Autodesk Fusion 360 part; units mm, degrees
sketch "草图1" plane through (0, 0, 0) normal (0, 0, 1) x (1, 0, 0)
  circle A0 centre (0, 0) radius 14.1
  line L0 (0, 9.064) -> (-7.85, -4.5326)
  line L1 (-7.85, -4.5326) -> (7.85, -4.5326)
  line L2 (7.85, -4.5326) -> (0, 9.064)
  line L3 (0, 9.064) -> (15.7, 9.064) construction
  circle A1 centre (0, 9.064) radius 1.5
  circle A2 centre (-7.85, -4.5326) radius 1.5
  circle A3 centre (7.85, -4.5326) radius 1.5
  point P0 (0, -0.0004)
  dimension "d1" = 28.2
  dimension "d2" = 15.7
  dimension "d3" = 120
  dimension "d4" = 9.064
  dimension "d5" = 3
  dimension "d6" = 3
  dimension "d7" = 3
extrude "拉伸1" add sketch "草图1" along normal blind 2 contours A0 | L0 L1 L2 A1 A2 A3
sketch "草图2" plane through (0, 0, 2) normal (0, 0, 1) x (-1, 0, 0)
  circle A0 centre (7.85, 4.5326) radius 1.5
  circle A1 centre (-7.85, 4.5326) radius 1.5
  circle A2 centre (0, -9.064) radius 1.5
  circle A3 centre (0, 0) radius 14.1
  circle A4 centre (0, 0) radius 2.2
  circle A5 centre (0, 0) radius 12
  circle A6 centre (0, 0) radius 4.2
  line L0 (0, 0) -> (4.5287, -11.1127)
  line L1 (0, 0) -> (11.7731, 2.3225)
  line L2 (0, 0) -> (7.3595, 9.4783)
  line L3 (0, 0) -> (-7.8979, 9.0345)
  line L4 (0, 0) -> (-11.8882, 1.6344)
  line L5 (0, 0) -> (-3.8752, -11.3571)
  dimension "d10" = 4.4
  dimension "d13" = 24
  dimension "d14" = 8.4
  dimension "d16" = 360
extrude "拉伸2" cut sketch "草图2" against normal blind 8 contours A4 L0 L1 | A4 L1 L2 | A4 L0 L5 | A4 L2 L3 | A4 L3 L4 | A4 L4 L5 | A5 A6 L0 L1 | A5 A6 L2 L3 | A5 A6 L4 L5
fillet "圆角1" radius 3 12 edges at (-1.585, 3.8894, 1) (-4.1206, -0.8129, 1) (-2.5758, -3.3174, 1) (2.7643, -3.1621, 1) (4.1609, -0.572, 1) (1.3563, 3.975, 1) (3.8752, 11.3571, 1) (11.8882, -1.6344, 1) (-4.5287, 11.1127, 1) (-11.7731, -2.3225, 1) (-7.3595, -9.4783, 1) (7.8979, -9.0345, 1)
Geometry check sheet. Reference: the model listing, model coordinates, mm. Give positions to 0.01 mm unless a question says otherwise; leave off trailing zeros. Write each loop counter-clockwise with the first axis right and the second up, starting at its lowest first coordinate (ties: lowest second). Pieces come first, ordered by that corner, then holes. Notation, with made-up numbers: (53.25, 11.5) -> (64.25, 11.5) arc R12 ccw to (64.25, 15.5) -> close; hole circle Ø3 at (56, 17.25). An arc over 180 degrees is marked (long way). One line per question, with ' | ' between items.
Item 1: Depth check by flat-ended pin: pin 1 (1 mm diameter, centred on y = -6, z = 1, fed in from -X); pin 2 (1.8 mm diameter, centred on x = 0, y = 9.064, fed in from +Z). Enter the tip coordinate at first touch or a pass-through.
Determined:
pin 1: x = -12.98 | pin 2: through
Item 2: Scan lines: line 1 along Y through (x, z) = (0, 0.4); line 2 along Y through (x, z) = (3, 0.95); line 3 along Y through (x, z) = (-7.85, 0.6). Record each from-to range of solid material in increasing order.
Determined:
line 1: -14.1 to -12, -4.2 to -2.2, 2.2 to 7.56, 10.56 to 14.1 | line 2: -13.78 to -11.62, -4.06 to 2.94, 8.59 to 13.78 | line 3: -11.71 to -6.03, -3.03 to -1.55, 9.07 to 11.71
Item 3: Sectioned sample at C-C, the plane z = 1.7. State how many separate pieces and enclosed holes the cut face has, plus the area to 3 significant figures.
Determined:
separate pieces: 1 | enclosed holes: 7 | area: 351 mm^2
Item 4: Sectioned sample at D-D, the plane x = 7.85. Record the boundary of the cut face in (y, z), plus the area to 3 significant figures.
Determined:
outline: (-11.71, 0) -> (-6.03, 0) -> (-6.03, 2) -> (-11.71, 2) -> close; (-3.03, 0) -> (-1.08, 0) -> (-1.08, 2) -> (-3.03, 2) -> close; (9.08, 0) -> (11.71, 0) -> (11.71, 2) -> (9.08, 2) -> close | area: 20.5 mm^2
Item 5: Sectioned sample at B-B, the plane y = 4. Record the boundary of the cut face in (x, z), plus the area to 3 significant figures.
Determined:
outline: (-13.52, 0) -> (-11.31, 0) -> (-11.31, 2) -> (-13.52, 2) -> close; (-2.4, 0) -> (2.21, 0) -> (2.21, 2) -> (-2.4, 2) -> close; (11.31, 0) -> (13.52, 0) -> (13.52, 2) -> (11.31, 2) -> close | area: 18.0 mm^2
Item 6: Sectioned sample at A-A, the plane x = 0. Record the boundary of the cut face in (y, z), plus the area to 3 significant figures.
Determined:
outline: (-14.1, 0) -> (-12, 0) -> (-12, 2) -> (-14.1, 2) -> close; (-4.2, 0) -> (-2.2, 0) -> (-2.2, 2) -> (-4.2, 2) -> close; (2.2, 0) -> (7.56, 0) -> (7.56, 2) -> (2.2, 2) -> close; (10.56, 0) -> (14.1, 0) -> (14.1, 2) -> (10.56, 2) -> close | area: 26.0 mm^2
